```python
from build123d import *

# Parameters (mm, degrees)
SKETCH1_R           = 1.5
BOSS_EXTRUDE1_DEPTH = 1.3
SKETCH3_R           = 8.460587883
CUT_EXTRUDE1_DEPTH  = 20


with BuildPart() as part:
    # Sketch1 → Boss-Extrude1 (new body)
    with BuildSketch(Plane.XY):
        Polygon((-29.648967954, 62.034735519), (-29.648967954, 1.034735519), (-10.648967954, -17.965264481), (50.351032046, -17.965264481), (69.351032046, 1.034735519), (69.351032046, 62.034735519), (50.351032046, 81.034735519), (-10.648967954, 81.034735519), align=None)
        with Locations((-1.648967954, 31.534735519)):
            Circle(SKETCH1_R, mode=Mode.SUBTRACT)
        with Locations((41.351032046, 31.534735519)):
            Circle(SKETCH1_R, mode=Mode.SUBTRACT)
        with Locations((41.351032046, 16.534735519)):
            Circle(SKETCH1_R, mode=Mode.SUBTRACT)
        with Locations((50.351032046, 16.534735519)):
            Circle(SKETCH1_R, mode=Mode.SUBTRACT)
    extrude(amount=BOSS_EXTRUDE1_DEPTH)

    # Sketch3 → Cut-Extrude1 (cut)
    with BuildSketch(Plane.XY.offset(1.3)):
        with Locations((20.92010377, 52.605401567)):
            Circle(SKETCH3_R)
    extrude(amount=-CUT_EXTRUDE1_DEPTH, mode=Mode.SUBTRACT)


solid = part.part
```
Design review of the part built by this model. Coordinates are the model's own, in mm. Give positions to 0.01 mm unless a question says otherwise; leave off trailing zeros. Write each loop counter-clockwise with the first axis right and the second up, starting at its lowest first coordinate (ties: lowest second). Pieces come first, ordered by that corner, then holes. Notation, with made-up numbers: (12, 72.25) -> (31, 72.25) arc R24 ccw to (31, 93.25) -> close; hole circle Ø6 at (66.5, -10). An arc over 180 degrees is marked (long way). Answer in a Markdown table with one row per item.
(1) To check wall thickness, follow probe 1 along X at (y, z) = (52, 0.85); probe 2 along X at (y, z) = (32.5, 0.35); probe 3 along Y at (x, z) = (22.5, 1.2). State the ranges of each line that lie inside material, in increasing order.
Results:
| item | result |
|---|---|
| probe 1 | -29.65 to 12.48, 29.36 to 69.35 |
| probe 2 | -29.65 to -2.8, -0.5 to 40.2, 42.5 to 69.35 |
| probe 3 | -17.97 to 44.29, 60.92 to 81.03 |
(2) Consider section C-C (x = 25.5). State the section outline as (y, z) points.
Results:
| item | result |
|---|---|
| outline | (-17.97, 0) -> (45.49, 0) -> (45.49, 1.3) -> (-17.97, 1.3) -> close; (59.72, 0) -> (81.03, 0) -> (81.03, 1.3) -> (59.72, 1.3) -> close |
(3) Consider section A-A (y = 58.5). State the section outline as (x, z) points, then the cut area to 3 significant figures.
Results:
| item | result |
|---|---|
| outline | (-29.65, 0) -> (14.85, 0) -> (14.85, 1.3) -> (-29.65, 1.3) -> close; (26.99, 0) -> (69.35, 0) -> (69.35, 1.3) -> (26.99, 1.3) -> close |
| area | 113 mm2 |
(4) Mouldability with a two-part tool opening along X and no side actions: class faces 1 (the cylindrical face through (39.852, 16.601, 0.641)), 2 (the flat face through (19, 32, 1.3)), 3 (the flat face through (-20.282, -8.332, 0.641)) as +X half, -X half, draft (parallel to the pull), parting line (faces both ways), or undercut.
Results:
| item | result |
|---|---|
| face 1 | undercut |
| face 2 | draft |
| face 3 | -X half |
(5) Consider section D-D (y = -9.5). State the section outline as (x, z) points.
Results:
| item | result |
|---|---|
| outline | (-19.11, 0) -> (58.82, 0) -> (58.82, 1.3) -> (-19.11, 1.3) -> close |
(6) Consider section B-B (z = 0.8). State the section outline as (x, y) points.
Results:
| item | result |
|---|---|
| outline | (-29.65, 1.03) -> (-10.65, -17.97) -> (50.35, -17.97) -> (69.35, 1.03) -> (69.35, 62.03) -> (50.35, 81.03) -> (-10.65, 81.03) -> (-29.65, 62.03) -> close; hole circle Ø3 at (-1.65, 31.53); hole circle Ø16.92 at (20.92, 52.61); hole circle Ø3 at (41.35, 16.53); hole circle Ø3 at (41.35, 31.53); hole circle Ø3 at (50.35, 16.53) |
